Design review of the part shown in the three views and the two pictorial views. Dimensions are in mm from the part's minimum x, y and z. Give positions to 0.01 mm unless a question says otherwise; leave off trailing zeros. Order: outer loops, then holes, each group sorted by start corner. A loop starts at its lowest first (then second) coordinate and runs counter-clockwise, first axis right, second up.
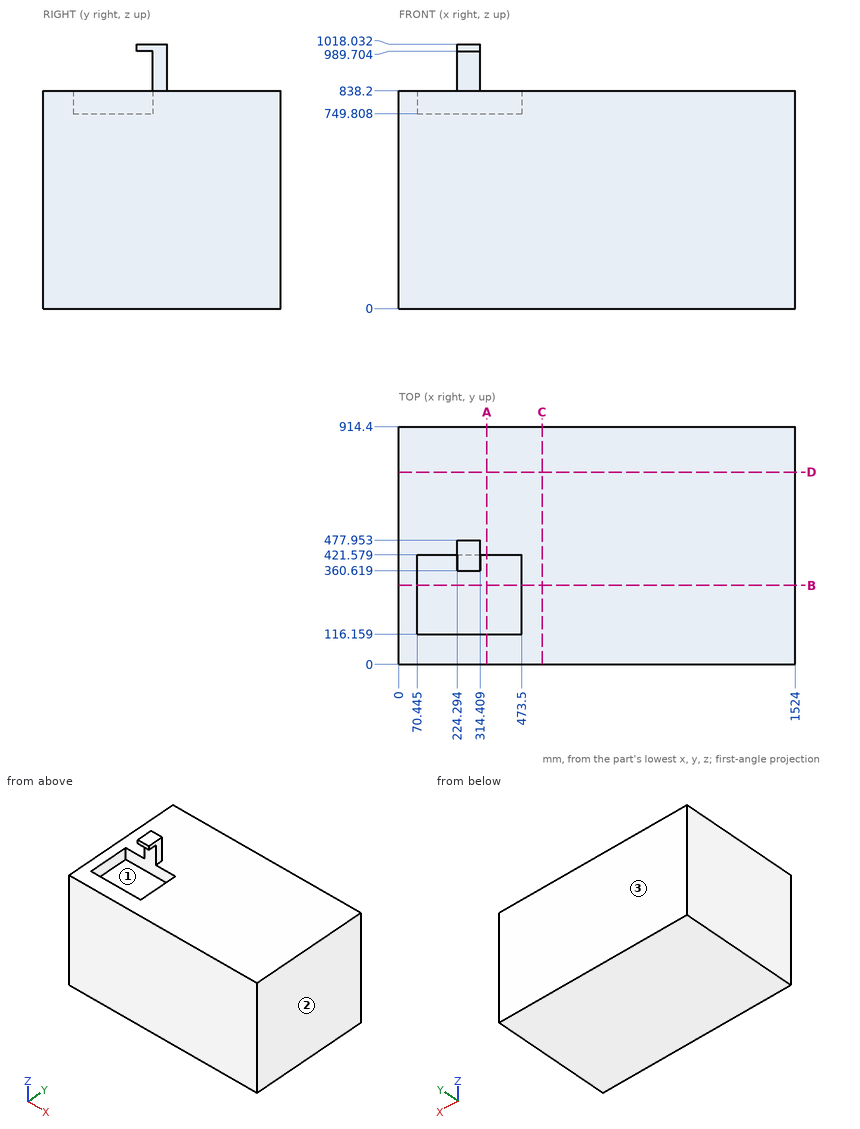
Item 1: Take a section at A-A (x = 338.5). Give the boundary of the cut face in (y, z).
Values found:
outline: (0, 0) - (914.4, 0) - (914.4, 838.2) - (421.58, 838.2) - (421.58, 749.81) - (116.16, 749.81) - (116.16, 838.2) - (0, 838.2) - close
Item 2: Take a section at D-D (y = 740). Give the boundary of the cut face in (x, z).
Values found:
outline: (0, 0) - (1524, 0) - (1524, 838.2) - (0, 838.2) - close
Item 3: Draft analysis for pull direction Y (two halves, no side actions). For the marked faces 1, 2 and 3, state which applies: released by +Y, released by -Y, zero draft, split by the parting line, or undercut.
Values found:
face 1: undercut
face 2: zero draft
face 3: released by +Y
Item 4: Clearance check with flat-ended pins moving along their axes: pin 1 Ø10 at (x, z) = (413.5, 820.5) entering from -Y; pin 2 Ø1 at (x, y) = (476, 560.5) entering from +Z; pin 3 Ø3 at (x, y) = (468, 415.5) entering from +Z; pin 4 Ø14 at (x, z) = (255.5, 997) entering from -Y. State where each tip first meets the part, or that it passes through.
Values found:
pin 1: stops at y = 0
pin 2: stops at z = 838.2
pin 3: stops at z = 749.81
pin 4: stops at y = 360.62
Item 5: For line 1 (X direction, y = 283, z = 825) (1 decimal); line 2 (Z direction, x = 445, y = 582.5); line 3 (Z direction, x = 447, y = 248.5), list the stretches that pass through material, from the lowest coordinate up.
Values found:
line 1: x = 0 to 70.4, 473.5 to 1524
line 2: z = 0 to 838.2
line 3: z = 0 to 749.81
Item 6: Take a section at C-C (x = 551). Give the boundary of the cut face in (y, z), and give its area (3 significant figures).
Values found:
outline: (0, 0) - (914.4, 0) - (914.4, 838.2) - (0, 838.2) - close
area: 766,000 mm2
Item 7: Take a section at B-B (y = 304). Give the boundary of the cut face in (x, z) (1 decimal).
Values found:
outline: (0, 0) - (1524, 0) - (1524, 838.2) - (473.5, 838.2) - (473.5, 749.8) - (70.4, 749.8) - (70.4, 838.2) - (0, 838.2) - close
